Design review of the part built by this model. Coordinates are the model's own, in mm. A direction names the side the tool comes from. Give positions to 0.01 mm unless a question says otherwise; leave off trailing zeros. Write each loop counter-clockwise with the first axis right and the second up, starting at its lowest first coordinate (ties: lowest second). Pieces come first, ordered by that corner, then holes. Notation, with made-up numbers: (51, -29) -> (89, -29) arc R21 ccw to (89, -13) -> close; hole circle Ø11 at (61.5, 18.25). An arc over 180 degrees is marked (long way). Answer as a JSON object with one key per item and string values.
```python
from build123d import *

# Parameters (mm, degrees)
F0_R     = 1.75
F1_DEPTH = 14
F2_DEPTH = 5
F3_R     = 2
F4_R     = 2.75
F5_DEPTH = 3
F6_R     = 1.75
F7_DEPTH = 2.5


with BuildPart() as f1:
    # F0 (on Top) → F1 (new body)
    with BuildSketch(Plane.XY):
        with BuildLine():
            Line((21.7761647301, 1.3240322888), (26.4237447456, 1.3240322888))
            ThreePointArc((26.4237447456, 1.3240322888), (27.5325816725, 4.2198246066), (25.8684580679, 6.8362773785))
            ThreePointArc((25.8684580679, 6.8362773785), (21.3298830229, 5.9305348281), (21.7761647301, 1.3240322888))
        make_face()
        with Locations((24.0999547378, 3.8740322888)):
            Circle(F0_R, mode=Mode.SUBTRACT)
    extrude(amount=-F1_DEPTH)



with BuildPart() as f1b:
    # F0 (on Top) → F1, piece 2 (new body)
    with BuildSketch(Plane.XY):
        with BuildLine():
            Line((26.0698554789, -17.7082796768), (26.0698554789, -12.0436557456))
            ThreePointArc((26.0698554789, -12.0436557456), (25.4051734809, -11.6823954116), (24.6777322905, -11.4746924945))
            Line((24.6777322905, -11.4746924945), (24.6851897334, -11.430791835))
            Line((24.6851897334, -11.430791835), (23.9175727699, -11.430791835))
            ThreePointArc((23.9175727699, -11.430791835), (20.8364414099, -15.9948871713), (26.0698554789, -17.7082796768))
        make_face()
        with Locations((24.0999547378, -14.8759677112)):
            Circle(F0_R, mode=Mode.SUBTRACT)
        with BuildLine():
            ThreePointArc((26.0698554789, -17.7082796768), (27.5499547378, -14.8759677112), (26.0698554789, -12.0436557456))
            Line((26.0698554789, -12.0436557456), (26.0698554789, -17.7082796768))
        make_face()
    extrude(amount=-F1_DEPTH)


with BuildPart() as f1_1:
    add(f1.part)

    add(f1b.part)  # F2 merges F1b
    # F0 (on Top) → F2 (join)
    with BuildSketch(Plane.XY):
        with BuildLine():
            Line((26.0698554789, -12.0436557456), (25.9312466019, 0.9501871991))
            ThreePointArc((25.9312466019, 0.9501871991), (26.1858877133, 1.1260541917), (26.4237447456, 1.3240322888))
            Line((26.4237447456, 1.3240322888), (21.7761647301, 1.3240322888))
            ThreePointArc((21.7761647301, 1.3240322888), (21.3298830229, 5.9305348281), (25.8684580679, 6.8362773785))
            Line((25.8684580679, 6.8362773785), (25.8227194135, 11.1240322888))
            Line((25.8227194135, 11.1240322888), (9.3227194135, 11.1240322888))
            Line((9.3227194135, 11.1240322888), (4.3655936032, 6.9737100091))
            Line((4.3655936032, 6.9737100091), (4.3655936032, -18.8759677112))
            Line((4.3655936032, -18.8759677112), (9.8819473522, -18.8759677112))
            Line((9.8819473522, -18.8759677112), (9.9476614486, -18.8759677112))
            Line((9.9476614486, -18.8759677112), (23.5200859606, -18.8759677112))
            Line((23.5200859606, -18.8759677112), (26.0698554789, -18.8759677112))
            Line((26.0698554789, -18.8759677112), (26.0698554789, -17.7082796768))
            ThreePointArc((26.0698554789, -17.7082796768), (20.8364414099, -15.9948871713), (23.9175727699, -11.430791835))
            Line((23.9175727699, -11.430791835), (24.6851897334, -11.430791835))
            Line((24.6851897334, -11.430791835), (24.6777322905, -11.4746924945))
            ThreePointArc((24.6777322905, -11.4746924945), (25.4051734809, -11.6823954116), (26.0698554789, -12.0436557456))
        make_face()
        with Locations((9.0999547378, -14.8759677112)):
            Circle(F0_R, mode=Mode.SUBTRACT)
        with Locations((9.0999547378, 3.8740322888)):
            Circle(F0_R, mode=Mode.SUBTRACT)
    extrude(amount=-F2_DEPTH)

    # F3
    f3_edges = [f1_1.edges().sort_by_distance(p)[0] for p in [
        (9.322719, 11.124032, -2.5),
        (4.365594, 6.97371, -2.5),
        (4.365594, -18.875968, -2.5),
        (25.822719, 11.124032, -2.5),
    ]]
    fillet(f3_edges, radius=F3_R)

    # F4 (on face) → F5 (cut)
    with BuildSketch(Plane.XY):
        with BuildLine():
            ThreePointArc((25.1289665719, 1.3240322888), (26.379519606, 2.3359536637), (26.8500410169, 3.8742895704))
            ThreePointArc((26.8500410169, 3.8742895704), (22.5617051102, 6.1537681595), (23.0711154619, 1.3240322888))
            Line((23.0711154619, 1.3240322888), (25.1289665719, 1.3240322888))
        make_face()
        with BuildLine():
            Line((25.1289665719, 1.3240322888), (23.0711154619, 1.3240322888))
            ThreePointArc((23.0711154619, 1.3240322888), (24.1000410169, 1.1242895704), (25.1289665719, 1.3240322888))
        make_face()
        with Locations((24.1000410169, -14.8761207238)):
            Circle(F4_R)
    extrude(amount=-F5_DEPTH, mode=Mode.SUBTRACT)

    # F6 (on face) → F7 (cut)
    with BuildSketch(Plane(origin=(0, 0, -5), x_dir=(1, 0, 0), z_dir=(0, 0, -1))):
        Polygon((10.6876679781, -1.1240322888), (7.5122414976, -1.1240322888), (5.9245282573, -3.8740322888), (7.5122414976, -6.6240322888), (10.6876679781, -6.6240322888), (12.2753812184, -3.8740322888), align=None)
        with Locations((9.0999547378, -3.8740322888)):
            Circle(F6_R, mode=Mode.SUBTRACT)
        Polygon((10.6876679781, 17.6259677112), (7.5122414976, 17.6259677112), (5.9245282573, 14.8759677112), (7.5122414976, 12.1259677112), (10.6876679781, 12.1259677112), (12.2753812184, 14.8759677112), align=None)
        with Locations((9.0999547378, 14.8759677112)):
            Circle(F6_R, mode=Mode.SUBTRACT)
    extrude(amount=-F7_DEPTH, mode=Mode.SUBTRACT)


solid = f1_1.part
```
(1) We need section A-A, the plane z = -10.5. State the section outline as (x, y) points, then the cut area to 3 significant figures.
Here are the results:
{"outline": "(21.78, 1.32) -> (26.42, 1.32) arc R3.45 ccw (long way) to start; (23.92, -11.43) arc R3.45 ccw (long way) to (24.68, -11.47) -> (24.69, -11.43) -> close; hole circle Ø3.5 at (24.1, -14.88); hole circle Ø3.5 at (24.1, 3.87)", "area": "52.7 mm²"}
(2) For line 1 along Y through (x, z) = (24, -1.25); line 2 along Y through (x, z) = (24.25, -12.75); line 3 along X through (y, z) = (-14.75, -8.25), list the stretches that pass through material, from the lowest coordinate up.
Here are the results:
{"line 1": "y = -18.88 to -17.62, -12.13 to 1.13, 6.62 to 11.12", "line 2": "y = -18.32 to -16.62, -13.13 to -11.43, 1.32 to 2.13, 5.62 to 7.32", "line 3": "x = 20.65 to 22.35, 25.85 to 27.55"}
(3) We need section B-B, the plane y = 3.25. State the section outline as (x, z) points (3 decimals).
Here are the results:
{"outline": "(4.366, -5) -> (6.285, -5) -> (6.285, -2.5) -> (7.465, -2.5) -> (7.465, 0) -> (4.366, 0) -> close; (10.735, -2.5) -> (11.915, -2.5) -> (11.915, -5) -> (20.707, -5) -> (20.707, -14) -> (22.465, -14) -> (22.465, -3) -> (21.422, -3) -> (21.422, 0) -> (10.735, 0) -> close; (25.735, -14) -> (27.493, -14) -> (27.493, 0) -> (26.778, 0) -> (26.778, -3) -> (25.735, -3) -> close"}
(4) We need section D-D, the plane x = 20.25. State the section outline as (y, z) points, then the cut area to 3 significant figures.
Here are the results:
{"outline": "(-18.88, -5) -> (11.12, -5) -> (11.12, 0) -> (-18.88, 0) -> close", "area": "150 mm²"}
(5) We need section C-C, the plane z = -4.25. State the section outline as (x, y) points.
Here are the results:
{"outline": "(4.37, -16.88) arc R2 ccw to (6.37, -18.88) -> (26.07, -18.88) -> (26.07, -17.71) arc R3.45 ccw to (26.07, -12.04) -> (25.93, 0.95) arc R3.45 ccw to (25.87, 6.84) -> (25.84, 9.15) arc R2 ccw to (23.84, 11.12) -> (10.05, 11.12) arc R2 ccw to (8.77, 10.66) -> (5.08, 7.57) arc R2 ccw to (4.37, 6.04) -> close; hole (5.92, -14.88) -> (7.51, -17.63) -> (10.69, -17.63) -> (12.28, -14.88) -> (10.69, -12.13) -> (7.51, -12.13) -> close; hole (5.92, 3.87) -> (7.51, 1.12) -> (10.69, 1.12) -> (12.28, 3.87) -> (10.69, 6.62) -> (7.51, 6.62) -> close; hole circle Ø3.5 at (24.1, -14.88); hole circle Ø3.5 at (24.1, 3.87)"}
(6) The part is to be moulded in two halves that separate along Y. For faces 1 (the cylindrical face through (4.97, -18.31, -2.54)), 2 (the flat face through (11.493, 2.518, -3.768)), 3 (the flat face through (11.493, -16.232, -3.768)), 4 (the flat face through (16, -4, 0)), say which applies: +Y half, -Y half, draft (parallel to the pull), parting line (faces both ways), or undercut.
Here are the results:
{"face 1": "-Y half", "face 2": "undercut", "face 3": "undercut", "face 4": "draft"}
(7) For faces 5 (the flat face through (26, 4, -3)), 6 (the flat face through (24, 1.324, -9)), 7 (the flat face through (6.707, -13.52, -3.768)), list the 3-axis set-ups (+Z, -Z, +X, -X, +Y, -Y) from which the entire face can be reached by the end or side of a thin tool; tool diameter is ignored.
Here are the results:
{"face 5": "+Z", "face 6": "-Z, +X, -X", "face 7": "-Z"}
(8) Clearance check with flat-ended pins moving along their axes: pin 1 (0.6 mm diameter, centred on x = 24, z = -10.5, fed in from +Y); pin 2 (1.2 mm diameter, centred on x = 8.5, z = -3.5, fed in from +Y); pin 3 (6 mm diameter, centred on x = 10, y = -13.5, fed in from -Z). State where each tip first meets the part, or that it passes through.
Here are the results:
{"pin 1": "stops at y = 7.32", "pin 2": "stops at y = 10.88", "pin 3": "stops at z = -5"}
